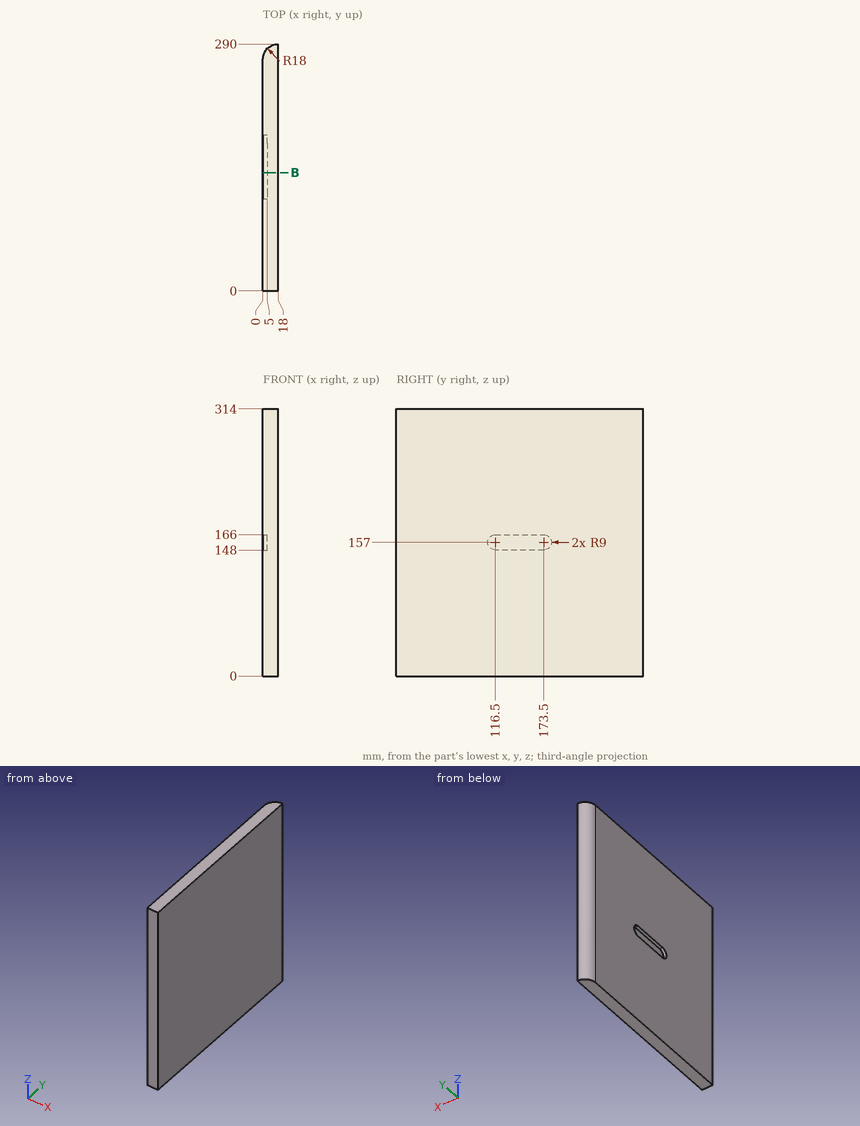
Study the drawing (mm; zero at the part's minimum x, y, z) and answer. Coordinates: 2 decimals unless noted, no trailing zeros. Order: outer loops, then holes, each group sorted by start corner. A loop starts at its lowest first (then second) coordinate and runs counter-clockwise, first axis right, second up. Notation, with made-up numbers: (28.5, 47) -> (83.5, 47) arc R20 ccw to (83.5, 55) -> close; hole circle Ø10 at (35.25, 10.25). An arc over 180 degrees is marked (long way). Answer in a Markdown table with one row per item. Add a question column.
Item 1: Each of these flat-tipped pins is pushed along its axis until it touches: P1, Ø3, axis at x = 4.5, z = 141, coming from the +Y side; P2, Ø1.5, axis at x = 2.5, y = 135.5, coming from the -Z side; P3, Ø5.5, axis at y = 128.5, z = 161, coming from the -X side; P4, Ø4, axis at x = 11, z = 225.5, coming from the +Y side. Where does it stop, or does it pass through?
Item 2: Find the intervals of material crossed by L1, parallel to X at y = 169, z = 154; L2, parallel to Y at x = 17, z = 113.5; L3, parallel to Z at x = 1.75, y = 181 (3 decimals), in increasing order. Write a range as from..to.
Item 3: Find section B-B (y = 139). Write down the section's boundary in (x, z).
Result set:
| question | item | result |
|---|---|---|
| 1 | P1 | stops at y = 285.42 |
| 1 | P2 | stops at z = 0 |
| 1 | P3 | stops at x = 5 |
| 1 | P4 | stops at y = 289.29 |
| 2 | L1 | x = 5..18 |
| 2 | L2 | y = 0..289.97 |
| 2 | L3 | z = 0..152.025, 161.975..314 |
| 3 | outline | (0, 0) -> (18, 0) -> (18, 314) -> (0, 314) -> (0, 166) -> (5, 166) -> (5, 148) -> (0, 148) -> close |
